from build123d import *

# Parameters (mm, degrees)
SKETCH_1_W          = 70
SKETCH_1_H          = 25
EXTRUDE_1_DEPTH     = 8
SKETCH_2_W          = 41
SKETCH_2_H          = 21
CUT_EXTRUDE_1_DEPTH = 24
CUT_EXTRUDE_4_DEPTH = 39.016443811
EXTRUDE_START       = -8
SKETCH_5_W          = 7
SKETCH_5_H          = 25
EXTRUDE_2_DEPTH     = 24.1
SKETCH_9_W          = 7
SKETCH_9_H          = 13.5
CUT_EXTRUDE_3_DEPTH = 2
EXTRUDE_11_DEPTH    = 0.5
SKETCH_20_W         = 70
SKETCH_20_H         = 19
EXTRUDE_12_DEPTH    = 1
M4X0_7_3_D          = 3.3


with BuildPart() as part:
    # 草圖1 → 填料-伸長1 (new body)
    with BuildSketch(Plane.XY):
        Rectangle(SKETCH_1_W, SKETCH_1_H)
    extrude(amount=EXTRUDE_1_DEPTH)

    # 草圖2 → 除料-伸長1 (cut)
    with BuildSketch(Plane(origin=(0, 0, 0), x_dir=(-1, 0, 0), z_dir=(0, 0, -1))):
        with Locations((0, -0.5)):
            Rectangle(SKETCH_2_W, SKETCH_2_H)
    extrude(amount=-CUT_EXTRUDE_1_DEPTH, mode=Mode.SUBTRACT)

    # 草圖10 → 除料-伸長4 (cut, through all)
    with BuildSketch(Plane.XY.offset(8)):
        with BuildLine():
            Line((-27, 0.5), (-14, 0.5))
            ThreePointArc((-14, 0.5), (-13, -0.5), (-14, -1.5))
            Line((-14, -1.5), (-27, -1.5))
            ThreePointArc((-27, -1.5), (-28, -0.5), (-27, 0.5))
        make_face()
    cut_extrude_4 = extrude(amount=-CUT_EXTRUDE_4_DEPTH, mode=Mode.SUBTRACT)

    # 草圖5 → 填料-伸長2 (add)
    with BuildSketch(Plane.XY.offset(8).offset(EXTRUDE_START)):
        with Locations((-31.5, 0)):
            Rectangle(SKETCH_5_W, SKETCH_5_H)
    extrude_2 = extrude(amount=-EXTRUDE_2_DEPTH)

    # 草圖8 → M4x0.7 螺紋孔1 (revolve, cut)
    with BuildSketch(Plane(origin=(-31.5, 0, -24.1), x_dir=(0, 1, 0), z_dir=(1, 0, 0))):
        Polygon((0, 0), (0, 30.991420021), (1.65, 30), (1.65, 0), align=None)
    m4x0_7_1 = revolve(axis=Axis((-31.5, 0, -30.45), (0, 0, 1)), mode=Mode.SUBTRACT)

    # 鏡射1: 除料-伸長4, 填料-伸長2, M4x0.7 螺紋孔1 across plane
    add(cut_extrude_4.mirror(Plane(origin=(0, 0, 0), x_dir=(0, 0, 1), z_dir=(1, 0, 0))), mode=Mode.SUBTRACT)
    add(extrude_2.mirror(Plane(origin=(0, 0, 0), x_dir=(0, 0, 1), z_dir=(1, 0, 0))))
    add(m4x0_7_1.mirror(Plane(origin=(0, 0, 0), x_dir=(0, 0, 1), z_dir=(1, 0, 0))), mode=Mode.SUBTRACT)

    # 草圖9 → 除料-伸長3 (cut)
    with BuildSketch(Plane.XZ.offset(12.5)):
        with Locations((31.5, -17.35)):
            Rectangle(SKETCH_9_W, SKETCH_9_H)
        with Locations((-31.5, -17.35)):
            Rectangle(SKETCH_9_W, SKETCH_9_H)
    extrude(amount=-CUT_EXTRUDE_3_DEPTH, mode=Mode.SUBTRACT)

    # 草圖19 → 填料-伸長11 (add)
    with BuildSketch(Plane.XZ.offset(12.5)):
        Polygon((35, 8), (-35, 8), (-35, -10.6), (-28, -10.6), (-28, 0), (28, 0), (28, -10.6), (35, -10.6), align=None)
    extrude(amount=EXTRUDE_11_DEPTH)

    # 草圖20 → 填料-伸長12 (add)
    with BuildSketch(Plane.XZ.offset(13)):
        with Locations((0, -1.5)):
            Rectangle(SKETCH_20_W, SKETCH_20_H)
    extrude(amount=EXTRUDE_12_DEPTH)

    # M4x0.7 螺紋孔3 (through all)
    with Locations(Plane.XY.offset(8)):
        with Locations((25, -5.5), (-25, 4.5), (-25, -5.5), (25, 4.5)):
            Hole(M4X0_7_3_D / 2)


solid = part.part
Input: part model. Units: mm. Frame: model coordinates. A direction names the side the tool comes from. Give positions to 0.01 mm unless a question says otherwise; leave off trailing zeros. Write each loop counter-clockwise with the first axis right and the second up, starting at its lowest first coordinate (ties: lowest second). Pieces come first, ordered by that corner, then holes. Notation, with made-up numbers: M 81,26.5 L 134,26.5 A20 ccw 134,59.5 Z; hole C 26,51.5 d10. An arc over 180 degrees is marked long. Write item = value, one per line. Start each with the question number.
1) First-contact query: pin 1 Ø5.5 at (x, z) = (-10.5, -3.5) entering from +Y; pin 2 Ø3 at (x, y) = (-30, -12.5) entering from -Z; pin 3 Ø3 at (x, y) = (-31.5, 0) entering from -Z. Flat tips, straight axial feed; report the tip coordinate or a pass-through.
2) Cut plane A-A on z = -18.5. Return the cut outline in (x, y), then the cut area to 3 significant figures.
3) Material intervals for line 1 along Y through (x, z) = (25, 2); line 2 along X through (y, z) = (0, -10.5); line 3 along X through (y, z) = (-3.25, -4.5), sorted ascending. Write a range as [from, to].
4) Cut plane C-C on y = -8. Return the cut outline in (x, z).
5) Draft query along X for faces 1 (the flat face through (-35, -1, -8)), 2 (the cylindrical face through (28, -0.5, 4.1)), 3 (the flat face through (20.5, -6, 4)), 4 (the flat face through (0, 12.5, 3)). Return one class per face: +X half, -X half, draft (parallel to the pull), parting line (faces both ways), or undercut.
6) Cut plane B-B on x = -9. Return the cut outline in (y, z), then the cut area to 3 significant figures.
7) Cut plane D-D on z = -2. Return the cut outline in (x, y), then the cut area to 3 significant figures.
8) Reachability of faces 5 (the conical face through (-31.2, 0.1, 6.7)), 6 (the flat face through (0, -11, 4)), 7 (the flat face through (0, -12, 0)) from +Z, -Z, +X, -X, +Y, -Y: full face, straight path, thin tool, end or side. Return the list, or none.
Solved:
q1.pin_1 = -13
q1.pin_2 = -11
q1.pin_3 = 5.99
q2.outline = M -35,-10.5 L -28,-10.5 L -28,12.5 L -35,12.5 Z; M 28,-10.5 L 35,-10.5 L 35,12.5 L 28,12.5 Z; hole C -31.5,0 d3.3; hole C 31.5,0 d3.3
q2.area = 305 mm2
q3.line_1 = [-14, -7.15], [-3.85, -1.5], [0.5, 2.85], [6.15, 12.5]
q3.line_2 = [-35, -33.15], [-29.85, -28], [28, 29.85], [33.15, 35]
q3.line_3 = [-35, -28], [28, 35]
q4.outline = M -35,-24.1 L -28,-24.1 L -28,0 L -20.5,0 L -20.5,8 L -35,8 Z; M 20.5,0 L 28,0 L 28,-24.1 L 35,-24.1 L 35,8 L 20.5,8 Z
q5.face_1 = -X half
q5.face_2 = undercut
q5.face_3 = undercut
q5.face_4 = draft
q6.outline = M -14,-11 L -13,-11 L -13,0 L -11,0 L -11,8 L -14,8 Z; M 10,0 L 12.5,0 L 12.5,8 L 10,8 Z
q6.area = 55.0 mm2
q7.outline = M -35,-14 L 35,-14 L 35,12.5 L 28,12.5 L 28,-13 L -28,-13 L -28,12.5 L -35,12.5 Z; hole C -31.5,0 d3.3; hole C 31.5,0 d3.3
q7.area = 410 mm2
q8.face_5 = -Z
q8.face_6 = +Z, -Z
q8.face_7 = -Z, +Y
